Answer from the drawing. Dimensions are ordinates in mm from the lowest x, y and z of the part. A direction names the side the tool comes from. Round coordinates to 2 decimals unless told otherwise and drop trailing zeros. Write each loop counter-clockwise with the first axis right and the second up, starting at its lowest first coordinate (ties: lowest second). Pieces come first, ordered by that corner, then holes. Notation, with made-up numbers: M -6,-28.75 L 43,-28.75 A24 ccw 43,-7.75 Z; hole C -4,43 d8. An arc over 180 degrees is marked long. One line per item, written item: value. Start each with the question number.
(1) Consider probe 1 along Z at (x, y) = (10.75, 18.75); probe 2 along X at (y, z) = (24.75, 11.5). Determine where each line is inside the solid, lowest interval first.
(2) Section C-C (x = 7) is taken. Determine the outline of the cut face in (y, z), plus the area to 3 significant figures.
(3) Section A-A (y = 10.5) is taken. Determine the outline of the cut face in (x, z), plus the area to 3 significant figures.
(4) Given P1, Ø4, axis at x = 9, z = 26.5, coming from the +Y side; P2, Ø11, axis at y = 24, z = 12.5, coming from the +X side; P3, Ø5, axis at x = 27, y = 15, coming from the +Z side; P4, Ø1.5, axis at y = 22.5, z = 15.5, coming from the +X side, each flat-ended and moving along its own axis, determine where each tip first touches the part or whether it passes through.
(5) For a pull along X with two mould halves and no side action, classify the marked faces 1, 2 and 3 as released by +X, released by -X, zero draft, split by the parting line, or undercut.
(6) Section D-D (y = 17) is taken. Determine the outline of the cut face in (x, z), plus the area to 3 significant figures.
(7) Section B-B (z = 13.5) is taken. Determine the outline of the cut face in (x, y).
(8) For the marked faces 4, 5, 6, 7 and 8, determine the directions among +Z, -Z, +X, -X, +Y, -Y from which every point of the face is accessible in a straight line to the end or side of a thin tool.
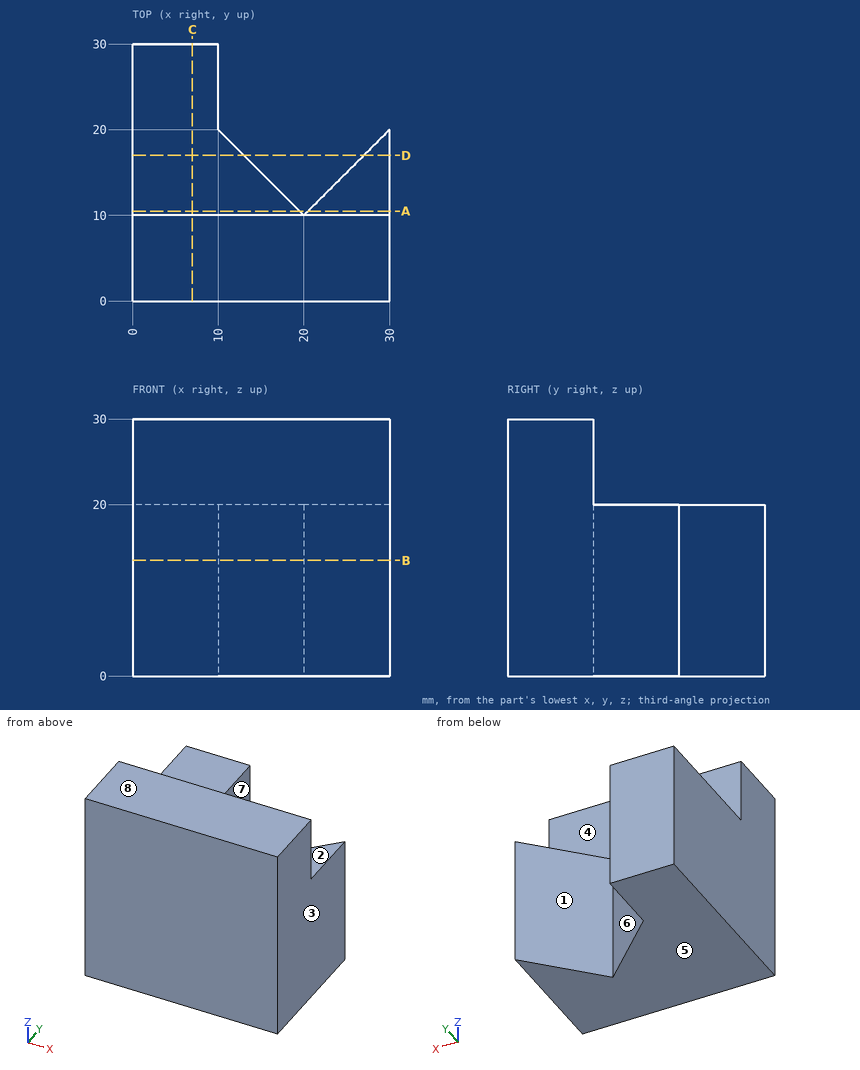
Recorded:
1. probe 1: z = 0 to 20
1. probe 2: x = 0 to 10
2. outline: M 0,0 L 30,0 L 30,20 L 10,20 L 10,30 L 0,30 Z
2. area: 700 mm2
3. outline: M 0,0 L 19.5,0 L 19.5,20 L 0,20 Z; M 20.5,0 L 30,0 L 30,20 L 20.5,20 Z
3. area: 580 mm2
4. P1: stops at y = 10
4. P2: stops at x = 30
4. P3: stops at z = 20
4. P4: stops at x = 10
5. face 1: undercut
5. face 2: zero draft
5. face 3: released by +X
6. outline: M 0,0 L 13,0 L 13,20 L 0,20 Z; M 27,0 L 30,0 L 30,20 L 27,20 Z
6. area: 320 mm2
7. outline: M 0,0 L 30,0 L 30,20 L 20,10 L 10,20 L 10,30 L 0,30 Z
8. face 4: +Z, +X, -X, +Y
8. face 5: -Z, +X, -X, +Y, -Y
8. face 6: +Z, -Z, +Y
8. face 7: +Z, -Z, +X, +Y
8. face 8: +Z, +X, -X, +Y, -Y
